```python
from build123d import *

# Parameters (mm, degrees)
SKETCH1_W           = 3
SKETCH1_H           = 2.8
BOSS_EXTRUDE1_DEPTH = 3


with BuildPart() as part:
    # Sketch1 → Boss-Extrude1 (new body)
    with BuildSketch(Plane(origin=(0, 0, 0), x_dir=(1, 0, 0), z_dir=(0, 1, 0))):
        Polygon((-10, -6.977624818), (-7, -6.977624818), (-7, -9.777624818), (7, -9.777624818), (7, -6.977624818), (10, -6.977624818), (10, -9.777624818), (13, -9.777624818), (13, 5.222375182), (10, 5.222375182), (10, 2.422375182), (7, 2.422375182), (7, 5.222375182), (-7, 5.222375182), (-7, 2.422375182), (-10, 2.422375182), (-10, 5.222375182), (-13, 5.222375182), (-13, -9.777624818), (-10, -9.777624818), align=None)
        with Locations((-8.5, -2.377624818)):
            Rectangle(SKETCH1_W, SKETCH1_H, mode=Mode.SUBTRACT)
        with Locations((8.5, -2.377624818)):
            Rectangle(SKETCH1_W, SKETCH1_H, mode=Mode.SUBTRACT)
    extrude(amount=BOSS_EXTRUDE1_DEPTH)


solid = part.part
```
Verification items for the finished model (mm, model axes). A direction names the side the tool comes from. Coordinates: 2 decimals unless noted, no trailing zeros. Order: outer loops, then holes, each group sorted by start corner. A loop starts at its lowest first (then second) coordinate and runs counter-clockwise, first axis right, second up. Notation, with made-up numbers: (13.25, 38) -> (69.25, 38) arc R25 ccw to (69.25, 70) -> close; hole circle Ø11 at (45, 60). An arc over 180 degrees is marked (long way). Put each result on its own line as item: value. Start each with the question number.
1) Go/stop test with flat-tipped pins: pin 1 (1.5 mm diameter, centred on x = -9, y = 1.5, fed in from +Z); pin 2 (0.9 mm diameter, centred on x = 9, y = 2, fed in from -Z). Record where each tip stops, or that it passes through.
2) Material ranges on L1, parallel to X at y = 1.5, z = -3.75; L2, parallel to Z at x = -8.75, y = 0.4, recorded low to high.
3) Cross-section at C-C (x = 7.75). Enter the section's corners in (y, z).
4) Cross-section at B-B (z = 8.25). Enter the section's corners in (x, y), plus the area to 3 significant figures.
5) Tool access check on faces 4 (the flat face through (-10, 1, 8)), 5 (the flat face through (8, 1, 0.978)), 6 (the flat face through (0, 3, 2)), 7 (the flat face through (13, 1, 2)), 8 (the flat face through (-8, 1, -2.422)). Record the directions out of +Z, -Z, +X, -X, +Y, -Y that give a thin tool (end or side, any length) a straight path to the whole face; none if there is none.
6) Release check for a two-part mould opening along Z. For faces 1 (the flat face through (7, 1, 8)), 2 (the flat face through (7, 1, 2)), 3 (the flat face through (8, 1, 6.978)) record: pulls with the +Z half, pulls with the -Z half, needs draft (parallel to the pull), parting line crosses it, or undercut.
7) Cross-section at A-A (y = 1.3). Enter the section's corners in (x, z).
Geometry check:
1. pin 1: stops at z = 6.98
1. pin 2: stops at z = -2.42
2. L1: x = -13 to -10, -7 to 7, 10 to 13
2. L2: z = -2.42 to 0.98, 3.78 to 6.98
3. outline: (0, -2.42) -> (3, -2.42) -> (3, 0.98) -> (0, 0.98) -> close; (0, 3.78) -> (3, 3.78) -> (3, 6.98) -> (0, 6.98) -> close
4. outline: (-13, 0) -> (-10, 0) -> (-10, 3) -> (-13, 3) -> close; (-7, 0) -> (7, 0) -> (7, 3) -> (-7, 3) -> close; (10, 0) -> (13, 0) -> (13, 3) -> (10, 3) -> close
4. area: 60.0 mm^2
5. face 4: +Z, +Y, -Y
5. face 5: +Y, -Y
5. face 6: +Z, -Z, +X, -X, +Y
5. face 7: +Z, -Z, +X, +Y, -Y
5. face 8: -Z, +Y, -Y
6. face 1: needs draft
6. face 2: undercut
6. face 3: pulls with the +Z half
7. outline: (-13, -5.22) -> (-10, -5.22) -> (-10, -2.42) -> (-7, -2.42) -> (-7, -5.22) -> (7, -5.22) -> (7, -2.42) -> (10, -2.42) -> (10, -5.22) -> (13, -5.22) -> (13, 9.78) -> (10, 9.78) -> (10, 6.98) -> (7, 6.98) -> (7, 9.78) -> (-7, 9.78) -> (-7, 6.98) -> (-10, 6.98) -> (-10, 9.78) -> (-13, 9.78) -> close; hole (-10, 0.98) -> (-7, 0.98) -> (-7, 3.78) -> (-10, 3.78) -> close; hole (7, 0.98) -> (10, 0.98) -> (10, 3.78) -> (7, 3.78) -> close
